Could you check a few things on this model? Use its own coordinates, in mm. Round coordinates to 2 decimals unless told otherwise and drop trailing zeros. Write each loop counter-clockwise with the first axis right and the second up, starting at its lowest first coordinate (ties: lowest second). Pieces come first, ordered by that corner, then holes.
```python
from build123d import *

# Parameters (mm, degrees)
SKETCH1_W           = 2.54
SKETCH1_H           = 2.54
BOSS_EXTRUDE1_DEPTH = 3
SKETCH2_R           = 0.66
BOSS_EXTRUDE2_DEPTH = 1.2
SKETCH4_R           = 0.3
CUT_EXTRUDE1_DEPTH  = 4
SKETCH3_R           = 0.23


with BuildPart() as part:
    # Sketch1 → Boss-Extrude1 (new body)
    with BuildSketch(Plane.XY):
        Rectangle(SKETCH1_W, SKETCH1_H)
    extrude(amount=BOSS_EXTRUDE1_DEPTH)

    # Sketch2 → Boss-Extrude2 (add)
    with BuildSketch(Plane(origin=(0, 0, 0), x_dir=(-1, 0, 0), z_dir=(0, 0, -1))):
        Circle(SKETCH2_R)
    extrude(amount=BOSS_EXTRUDE2_DEPTH)

    # Sketch4 → Cut-Extrude1 (cut)
    with BuildSketch(Plane.XY.offset(3)):
        Circle(SKETCH4_R)
    extrude(amount=-CUT_EXTRUDE1_DEPTH, mode=Mode.SUBTRACT)

    # Sweep1: sweep along a path in Sketch5
    with BuildLine(Plane(origin=(0, 0, 0), x_dir=(1, 0, 0), z_dir=(0, 1, 0))) as sweep1_path:
        Line((0, 1.2), (0, 1.6))
        ThreePointArc((0, 1.6), (0.292893219, 2.307106781), (1, 2.6))
        Line((1, 2.6), (4.47, 2.6))
    # Sketch3 → Sweep1 (sweep)
    with BuildSketch(Plane(origin=(0, 0, -1.2), x_dir=(-1, 0, 0), z_dir=(0, 0, -1))):
        Circle(SKETCH3_R)
    sweep(path=sweep1_path.line)


solid = part.part
```
Q1. Imagine slicing it at D-D, the plane y = 0.4. Write out the boundary of the cut face in (x, z), then the cut area to 3 significant figures.
Q2. Imagine slicing it at C-C, the plane x = 2. Write out the boundary of the cut face in (y, z), then the cut area to 3 significant figures.
Q3. Imagine slicing it at A-A, the plane z = 2. Write out the boundary of the cut face in (x, y).
Q4. Imagine slicing it at B-B, the plane y = 0. Write out the boundary of the cut face in (x, z), then the cut area to 3 significant figures.
Q5. If I drill on L1, parallel to Y at x = 0, z = 0.3; L2, parallel to Z at x = -0.85, y = -1.05; L3, parallel to X at y = 0.2, z = 0.35, over which ranges is the centre line in solid material (lowest first)?
Results found:
1. outline: (-1.27, 0) - (-0.52, 0) - (-0.52, -1.2) - (0.52, -1.2) - (0.52, 0) - (1.27, 0) - (1.27, 3) - (-1.27, 3) - close
1. area: 8.88 mm2
2. outline: circle Ø0.46 at (0, -2.6)
2. area: 0.166 mm2
3. outline: (-1.27, -1.27) - (1.27, -1.27) - (1.27, 1.27) - (-1.27, 1.27) - close; hole circle Ø0.6 at (0, 0)
4. outline: (-1.27, 0) - (-0.66, 0) - (-0.66, -1.2) - (-0.23, -1.2) - (-0.23, -1.6) arc R1.23 ccw to (1, -2.83) - (4.47, -2.83) - (4.47, -2.37) - (1, -2.37) arc R0.77 cw to (0.23, -1.6) - (0.23, -1.2) - (0.66, -1.2) - (0.66, 0) - (1.27, 0) - (1.27, 3) - (0.3, 3) - (0.3, -1) - (-0.3, -1) - (-0.3, 3) - (-1.27, 3) - close
4. area: 9.31 mm2
5. L1: y = -1.27 to -0.3, 0.3 to 1.27
5. L2: z = 0 to 3
5. L3: x = -1.27 to -0.22, 0.22 to 1.27
